Input: part model. Units: mm. Frame: model coordinates. Coordinates: 2 decimals unless noted, no trailing zeros. Write each loop counter-clockwise with the first axis right and the second up, starting at its lowest first coordinate (ties: lowest second). Pieces come first, ordered by that corner, then holes. Notation, with made-up numbers: M 82,88 L 136,88 A21 cw 136,115 Z; hole C 25,54 d8. An arc over 180 degrees is marked long. Write each question's results on one line, items separated by ' | '. Start each with the question number.
1. Ray query, probe 1 along Z at (x, y) = (-76.5, -24.5); probe 2 along X at (y, z) = (-52, -76); probe 3 along X at (y, z) = (-64, -65.5). Return the intervals inside material, ascending.
2. Pull-direction query (Z, two-part tool) for faces 1 (the cylindrical face through (-75.61, -74.67, -137.68)), 2 (the flat face through (-61, 0, -68)), 3 (the cylindrical face through (-66.1, -38.6, -68.5)), 4 (the flat face through (-112.712, -35.062, -24.944)); classes: +Z half, -Z half, draft (parallel to the pull), parting line (faces both ways), or undercut.
3. First-contact query: pin 1 (8 mm diameter, centred on y = -64.5, z = -107, fed in from +X); pin 2 (1.5 mm diameter, centred on y = -40.5, z = -106.5, fed in from +X); pin 3 (4 mm diameter, centred on y = -15, z = -120, fed in from +X); pin 4 (23 mm diameter, centred on x = -76.2, z = -76.2, fed in from +Y). Flat tips, straight axial feed; report the tip coordinate or a pass-through.
4. Section query A-A, the plane y = -60.5. Output: boundary loops of the cut face in (x, z), and give its area (3 significant figures).
```python
from build123d import *

# Parameters (mm, degrees)
F1_DEPTH     = 76.2
F2_R         = 5.08
F3_T1_DEPTH  = 80.3470901057
F3_T6_DEPTH  = 5.08
F5_T1_DEPTH  = 80.3470901057
F5_T6_DEPTH  = 5.08
F5_T12_DEPTH = 5.08
F6_T1_DEPTH  = 80.3470901057
F6_T6_DEPTH  = 5.08
F6_T12_DEPTH = 5.08
F7_D         = 25.4


# Not quite as in the source:
# - a fillet or chamfer that OpenCascade refuses, or shapes differently, is made with other operations: its cross-section is extruded or revolved along the edge and cut away or added
# - a feature of the source that left no trace in its solid (it failed there, or was rolled back) is left out


with BuildPart() as f1:
    # F0 (on Front) → F1 (new body)
    with BuildSketch(Plane.XZ):
        Polygon((-30.48, -139.1281814039), (-2.2234860344, -52.1635735539), (-76.2, 1.5835099157), (-150.1765139656, -52.1635735539), (-121.92, -139.1281814039), align=None)
    extrude(amount=F1_DEPTH)

    # F2
    f2_edges = [f1.edges().sort_by_distance(p)[0] for p in [
        (-16.351743, -76.2, -95.645877),
        (-39.211743, -76.2, -25.290032),
        (-113.188257, -76.2, -25.290032),
        (-136.048257, -76.2, -95.645877),
        (-76.2, -76.2, -139.128181),
    ]]
    fillet(f2_edges, radius=F2_R)

    # F3: fillet of radius 5.08 on 1 edges, made by hand

    # F3_s2 → F3_t1 (cut)
    with BuildSketch(Plane.XZ.offset(-9.2270901057)):
        with BuildLine():
            ThreePointArc((-149.0359829051, -55.6737672225), (-149.0359829051, -52.5341545596), (-147.190564884, -49.9941545596))
            Line((-147.190564884, -49.9941545596), (-150.1765139656, -52.1635735539))
            Line((-150.1765139656, -52.1635735539), (-149.0359829051, -55.6737672225))
        make_face()
    extrude(amount=F3_T1_DEPTH, mode=Mode.SUBTRACT)


with BuildPart() as f3_tool4:
    # F3_s5 → F3_t6 (new body)
    with BuildSketch(Plane.XZ.offset(71.12)):
        Polygon((-144.2046158024, -54.1039608911), (-149.0359829051, -55.6737672225), (-150.1765139656, -52.1635735539), (-147.190564884, -49.9941545596), align=None)
    extrude(amount=F3_T6_DEPTH)

    # F3_s7 → F3_t8 (revolve, cut)
    with BuildSketch(Plane(origin=(-144.2046158024, -71.12, -54.1039608911), x_dir=(0.9510565163, 0, -0.3090169944), z_dir=(-0.3090169944, 0, -0.9510565163))):
        with BuildLine():
            ThreePointArc((0, -5.08), (5.08, 0), (0, 5.08))
            Line((0, 5.08), (0, -5.08))
        make_face()
    revolve(axis=Axis((-144.2046158024, -71.12, -54.1039608911), (0, -1, 0)), mode=Mode.SUBTRACT)


with BuildPart() as f1_1:
    add(f1.part)

    # F3_t3: cut F3_tool4
    add(f3_tool4.part, mode=Mode.SUBTRACT)

    # F5: fillet of radius 5.08 on 2 edges, made by hand

    # F5_s2 → F5_t1 (cut)
    with BuildSketch(Plane.XZ.offset(-9.2270901057)):
        with BuildLine():
            ThreePointArc((-29.3394689395, -135.6179877354), (-31.1848869606, -138.1579877354), (-34.1708360423, -139.1281814039))
            Line((-34.1708360423, -139.1281814039), (-30.48, -139.1281814039))
            Line((-30.48, -139.1281814039), (-29.3394689395, -135.6179877354))
        make_face()
        with BuildLine():
            ThreePointArc((-3.3640170949, -55.6737672225), (-3.3640170949, -52.5341545596), (-5.209435116, -49.9941545596))
            Line((-5.209435116, -49.9941545596), (-2.2234860344, -52.1635735539))
            Line((-2.2234860344, -52.1635735539), (-3.3640170949, -55.6737672225))
        make_face()
    extrude(amount=F5_T1_DEPTH, mode=Mode.SUBTRACT)


with BuildPart() as f5_tool4:
    # F5_s5 → F5_t6 (new body)
    with BuildSketch(Plane.XZ.offset(71.12)):
        Polygon((-8.1953841976, -54.1039608911), (-3.3640170949, -55.6737672225), (-2.2234860344, -52.1635735539), (-5.209435116, -49.9941545596), align=None)
    extrude(amount=F5_T6_DEPTH)

    # F5_s7 → F5_t8 (revolve, cut)
    with BuildSketch(Plane(origin=(-8.1953841976, -71.12, -54.1039608911), x_dir=(-0.9510565163, 0, -0.3090169944), z_dir=(-0.3090169944, 0, 0.9510565163))):
        with BuildLine():
            ThreePointArc((0, -5.08), (5.08, 0), (0, 5.08))
            Line((0, 5.08), (0, -5.08))
        make_face()
    revolve(axis=Axis((-8.1953841976, -71.12, -54.1039608911), (0, -1, 0)), mode=Mode.SUBTRACT)


with BuildPart() as f1_2:
    add(f1_1.part)

    # F5_t3: cut F5_tool4
    add(f5_tool4.part, mode=Mode.SUBTRACT)


with BuildPart() as f5_tool10:
    # F5_s11 → F5_t12 (new body)
    with BuildSketch(Plane.XZ.offset(71.12)):
        Polygon((-34.1708360423, -134.0481814039), (-29.3394689395, -135.6179877354), (-30.48, -139.1281814039), (-34.1708360423, -139.1281814039), align=None)
    extrude(amount=F5_T12_DEPTH)

    # F5_s13 → F5_t14 (revolve, cut)
    with BuildSketch(Plane(origin=(-34.1708360423, -71.12, -134.0481814039), x_dir=(-0.5877852523, 0, 0.8090169944), z_dir=(0.8090169944, 0, 0.5877852523))):
        with BuildLine():
            ThreePointArc((0, -5.08), (5.08, 0), (0, 5.08))
            Line((0, 5.08), (0, -5.08))
        make_face()
    revolve(axis=Axis((-34.1708360423, -71.12, -134.0481814039), (0, -1, 0)), mode=Mode.SUBTRACT)


with BuildPart() as f1_3:
    add(f1_2.part)

    # F5_t9: cut F5_tool10
    add(f5_tool10.part, mode=Mode.SUBTRACT)

    # F6: fillet of radius 5.08 on 2 edges, made by hand

    # F6_s2 → F6_t1 (cut)
    with BuildSketch(Plane.XZ.offset(-9.2270901057)):
        with BuildLine():
            ThreePointArc((-79.1859490816, -0.5859090786), (-76.2, 0.38428459), (-73.2140509184, -0.5859090786))
            Line((-73.2140509184, -0.5859090786), (-76.2, 1.5835099157))
            Line((-76.2, 1.5835099157), (-79.1859490816, -0.5859090786))
        make_face()
        with BuildLine():
            ThreePointArc((-123.0605310605, -135.6179877354), (-121.2151130394, -138.1579877354), (-118.2291639577, -139.1281814039))
            Line((-118.2291639577, -139.1281814039), (-121.92, -139.1281814039))
            Line((-121.92, -139.1281814039), (-123.0605310605, -135.6179877354))
        make_face()
    extrude(amount=F6_T1_DEPTH, mode=Mode.SUBTRACT)


with BuildPart() as f6_tool4:
    # F6_s5 → F6_t6 (new body)
    with BuildSketch(Plane.XZ.offset(71.12)):
        Polygon((-118.2291639577, -134.0481814039), (-123.0605310605, -135.6179877354), (-121.92, -139.1281814039), (-118.2291639577, -139.1281814039), align=None)
    extrude(amount=F6_T6_DEPTH)

    # F6_s7 → F6_t8 (revolve, cut)
    with BuildSketch(Plane(origin=(-118.2291639577, -71.12, -134.0481814039), x_dir=(0.5877852523, 0, 0.8090169944), z_dir=(0.8090169944, 0, -0.5877852523))):
        with BuildLine():
            ThreePointArc((0, -5.08), (5.08, 0), (0, 5.08))
            Line((0, 5.08), (0, -5.08))
        make_face()
    revolve(axis=Axis((-118.2291639577, -71.12, -134.0481814039), (0, -1, 0)), mode=Mode.SUBTRACT)


with BuildPart() as f1_4:
    add(f1_3.part)

    # F6_t3: cut F6_tool4
    add(f6_tool4.part, mode=Mode.SUBTRACT)


with BuildPart() as f6_tool10:
    # F6_s11 → F6_t12 (new body)
    with BuildSketch(Plane.XZ.offset(71.12)):
        Polygon((-76.2, -4.69571541), (-79.1859490816, -0.5859090786), (-76.2, 1.5835099157), (-73.2140509184, -0.5859090786), align=None)
    extrude(amount=F6_T12_DEPTH)

    # F6_s13 → F6_t14 (revolve, cut)
    with BuildSketch(Plane(origin=(-76.2, -71.12, -4.69571541), x_dir=(0, 0, -1), z_dir=(-1, 0, 0))):
        with BuildLine():
            ThreePointArc((0, -5.08), (5.08, 0), (0, 5.08))
            Line((0, 5.08), (0, -5.08))
        make_face()
    revolve(axis=Axis((-76.2, -71.12, -4.69571541), (0, -1, 0)), mode=Mode.SUBTRACT)


with BuildPart() as f1_5:
    add(f1_4.part)

    # F6_t9: cut F6_tool10
    add(f6_tool10.part, mode=Mode.SUBTRACT)

    # F7 (through all)
    with Locations(Plane(origin=(0, 0, 0), x_dir=(1, 0, 0), z_dir=(0, 1, 0))):
        with Locations((-76.2, 76.2)):
            Hole(F7_D / 2)


solid = f1_5.part
```
Answer:
1) probe 1: -139.13 to -88.9, -63.5 to 0.38 | probe 2: -142.43 to -88.9, -63.5 to -9.97 | probe 3: -145.84 to -83.04, -69.36 to -6.56
2) face 1: -Z half | face 2: draft | face 3: undercut | face 4: +Z half
3) pin 1: x = -18.74 | pin 2: x = -19.63 | pin 3: x = -23.62 | pin 4: through
4) outline: M -149.04,-55.67 L -123.06,-135.62 A5.08 ccw -118.23,-139.13 L -34.17,-139.13 A5.08 ccw -29.34,-135.62 L -3.36,-55.67 A5.08 ccw -5.21,-49.99 L -73.21,-0.59 A5.08 ccw -79.19,-0.59 L -147.19,-49.99 A5.08 ccw Z; hole C -76.2,-76.2 d25.4 | area: 13,900 mm^2
